```python
from build123d import *

# Parameters (mm, degrees)
SKETCH_1_R          = 3.5
EXTRUDE_1_DEPTH     = 3.9
SKETCH_2_R          = 2
EXTRUDE_2_DEPTH     = 20
CUT_EXTRUDE_1_DEPTH = 2.4


with BuildPart() as part:
    # 草图1 → 凸台-拉伸1 (new body)
    with BuildSketch(Plane(origin=(0, 0, 0), x_dir=(1, 0, 0), z_dir=(0, 1, 0))):
        Circle(SKETCH_1_R)
    extrude(amount=EXTRUDE_1_DEPTH)

    # 草图2 → 凸台-拉伸2 (add)
    with BuildSketch(Plane(origin=(0, 3.9, 0), x_dir=(1, 0, 0), z_dir=(0, 1, 0))):
        Circle(SKETCH_2_R)
    extrude(amount=EXTRUDE_2_DEPTH)

    # 草图3 → 切除-拉伸1 (cut)
    with BuildSketch(Plane.XZ):
        Polygon((1.725, 0), (0.8625, 1.493893822), (-0.8625, 1.493893822), (-1.725, 0), (-0.8625, -1.493893822), (0.8625, -1.493893822), align=None)
    extrude(amount=-CUT_EXTRUDE_1_DEPTH, mode=Mode.SUBTRACT)


solid = part.part
```
The listing builds one solid part. Answer for the finished solid, in the listing's coordinates (mm). A direction names the side the tool comes from. Round coordinates to 2 decimals unless told otherwise and drop trailing zeros. Loops run counter-clockwise (first coordinate to the right, second up) from the corner with the lowest first, then second, coordinate; pieces in that order, holes last.
1) For faces 4 (the face through (2, 3.9, 2)), 5 (the face through (0, 0, 2)), 6 (the face through (-1.3, 1.18, -0.74)), determine the directions among +Z, -Z, +X, -X, +Y, -Y from which every point of the face is accessible in a straight line to the end or side of a thin tool.
Outcome:
face 4: +Y
face 5: +Z, -Z, +X, -X, -Y
face 6: -Y
2) A cutting plane is placed at C-C on z = -0.5. Determine the outline of the cut face in (x, y).
Outcome:
outline: (-3.46, 0) - (-1.44, 0) - (-1.44, 2.4) - (1.44, 2.4) - (1.44, 0) - (3.46, 0) - (3.46, 3.9) - (1.94, 3.9) - (1.94, 23.9) - (-1.94, 23.9) - (-1.94, 3.9) - (-3.46, 3.9) - close
3) Consider line 1 (X direction, y = 16.75, z = 0); line 2 (Y direction, x = -0.25, z = 0); line 3 (Y direction, x = -1.25, z = 1.75). Determine where each line is inside the solid, lowest interval first.
Outcome:
line 1: x = -2 to 2
line 2: y = 2.4 to 23.9
line 3: y = 0 to 3.9
4) A cutting plane is placed at A-A on x = 0. Determine the outline of the cut face in (y, z), plus the area to 3 significant figures.
Outcome:
outline: (0, -3.5) - (3.9, -3.5) - (3.9, -2) - (23.9, -2) - (23.9, 2) - (3.9, 2) - (3.9, 3.5) - (0, 3.5) - (0, 1.49) - (2.4, 1.49) - (2.4, -1.49) - (0, -1.49) - close
area: 100 mm2
5) Given P1, Ø1.5, axis at x = -2.5, y = 21, coming from the -Z side; P2, Ø1.5, axis at x = 1.5, y = 19.5, coming from the -Z side; P3, Ø2, axis at x = 1, y = 14.5, coming from the +Z side, each flat-ended and moving along its own axis, determine where each tip first touches the part or whether it passes through.
Outcome:
P1: stops at z = -0.97
P2: stops at z = -1.85
P3: stops at z = 2
6) A cutting plane is placed at D-D on x = 2.25. Determine the outline of the cut face in (y, z).
Outcome:
outline: (0, -2.68) - (3.9, -2.68) - (3.9, 2.68) - (0, 2.68) - close
7) For a pull along X with two mould halves and no side action, classify faces 1 (the face through (1.288, 1.183, -0.757)), 2 (the face through (0, 23.9, 0)), 3 (the face through (0, 14, 2)) as released by +X, released by -X, zero draft, split by the parting line, or undercut.
Outcome:
face 1: undercut
face 2: zero draft
face 3: split by the parting line
8) A cutting plane is placed at B-B on y = 6.75. Determine the outline of the cut face in (x, z), plus the area to 3 significant figures.
Outcome:
outline: circle Ø4 at (0, 0)
area: 12.6 mm2
